from build123d import *

# Parameters (mm, degrees)
F1_DEPTH = 48
F3_DEPTH = 20
F4_T     = 1.5


# Not quite as in the source:
# - a shell that OpenCascade refuses in one call is made with other operations: the cavity is built on its own and cut out


with BuildPart() as f1:
    # F0 (on Top) → F1 (new body)
    with BuildSketch(Plane.XY):
        Polygon((22.5, 22.8382229426), (-22.5, 22.8382229426), (-25, -9.1617770574), (25, -9.1617770574), align=None)
        Polygon((19, 39.8382229426), (-19, 39.8382229426), (-22.5, 22.8382229426), (22.5, 22.8382229426), align=None)
    extrude(amount=F1_DEPTH)

    # F2 (on face) → F3 (cut)
    with BuildSketch(Plane.XY.offset(48)):
        Polygon((22.5, 22.8382229426), (-22.5, 22.8382229426), (-25, -9.1617770574), (25, -9.1617770574), align=None)
    extrude(amount=-F3_DEPTH, mode=Mode.SUBTRACT)

    # F4: shell of thickness 1.5, made by hand


with BuildPart() as f4_core1:
    # F4_t2: copy of F1
    add(f1.part)

    # the walls: a layer under each face that stays
    f4_faces = [f4_core1.faces().sort_by_distance(p)[0] for p in [
        (0, 15.3382229426, 0),
        (23.75, 6.8382229426, 14),
        (-23.75, 6.8382229426, 14),
        (20.75, 31.3382229426, 24),
        (0, 39.8382229426, 24),
        (-20.75, 31.3382229426, 24),
        (0, 31.3382229426, 48),
    ]]
    thicken(f4_faces, amount=-F4_T, mode=Mode.SUBTRACT)


with BuildPart() as f1_1:
    add(f1.part)

    # what is left inside the walls is the cavity
    f4_cavity = [f4_core1.part.solids().sort_by_distance(p)[0] for p in [
        (0, 6.671556, 1.515),
    ]]
    add(f4_cavity, mode=Mode.SUBTRACT)


solid = f1_1.part
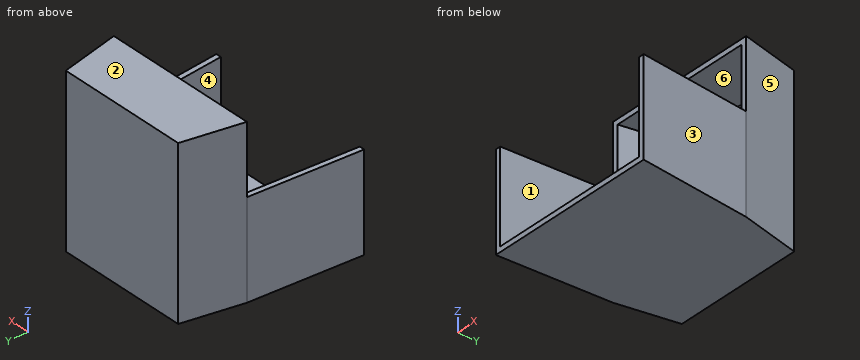
Could you check a few things on this model? Use its own coordinates, in mm. Face numbers are marked on the shaded views. A direction names the side the tool comes from. Give positions to 0.01 mm unless a question says otherwise; leave off trailing zeros. Write each loop counter-clockwise with the first axis right and the second up, starting at its lowest first coordinate (ties: lowest second). Pieces come first, ordered by that corner, then holes. Notation, with made-up numbers: (-39.5, 3) -> (-24.5, 3) arc R29 ccw to (-24.5, 23) -> close; hole circle Ø10 at (-3, 22). An arc over 180 degrees is marked (long way). Write each question's results on one line, items separated by ' | '. Start each with the question number.
Q1. Suppose I cut it at D-D, the plane y = 14. List the corners of the cut face in (x, z) for me.
Q2. Suppose I cut it at A-A, the plane x = -7. List the corners of the cut face in (y, z) for me, and give its area (4 significant figures).
Q3. Suppose I cut it at B-B, the plane y = 28.5. List the corners of the cut face in (x, z) for me, and give its area (3 significant figures).
Q4. Suppose I cut it at C-C, the plane z = 18. List the corners of the cut face in (x, y) for me, and give its area (3 significant figures).
Q5. Which directions (+Z, -Z, +X, -X, +Y, -Y) give clear straight access to the entire face, cutting with the end or side of a thin tool? Please do the marked faces 5 and 6.
Q6. We'd pull the mould along X, two halves only. Please class the marked faces 1, 2, 3 and 4: +X half, -X half, draft (parallel to the pull), parting line (faces both ways), or undercut.
Q7. I'm going to push flat-ended pins straight in: pin 1 Ø3 at (x, z) = (8, 33.5) entering from -Y; pin 2 Ø3 at (x, y) = (22.5, 14) entering from +Z; pin 3 Ø22 at (x, z) = (1.5, 38) entering from -Y. Where does each tip first touch, or does it pass through?
Q8. I need wall thicknesses on probe 1 along Z at (x, y) = (0, 35); probe 2 along Y at (x, z) = (-15, 31.5); probe 3 along X at (y, z) = (34.5, 23.5). Which ranges of each line are inside material? Lowest first, please.
Outcome:
1) outline: (-23.19, 0) -> (23.19, 0) -> (23.19, 28) -> (21.69, 28) -> (21.69, 1.5) -> (-21.69, 1.5) -> (-21.69, 28) -> (-23.19, 28) -> close
2) outline: (-9.16, 0) -> (39.84, 0) -> (39.84, 48) -> (22.84, 48) -> (22.84, 46.5) -> (38.34, 46.5) -> (38.34, 1.5) -> (-9.16, 1.5) -> close | area: 166.5 mm2
3) outline: (-21.33, 0) -> (21.33, 0) -> (21.33, 48) -> (-21.33, 48) -> close; hole (-19.8, 1.5) -> (19.8, 1.5) -> (19.8, 46.5) -> (-19.8, 46.5) -> close | area: 266 mm2
4) outline: (-25, -9.16) -> (-23.5, -9.16) -> (-21.01, 22.63) -> (-17.78, 38.34) -> (17.78, 38.34) -> (21.01, 22.63) -> (23.5, -9.16) -> (25, -9.16) -> (22.5, 22.84) -> (19, 39.84) -> (-19, 39.84) -> (-22.5, 22.84) -> close | area: 201 mm2
5) face 5: +Z, -Z, +X, +Y | face 6: -Y
6) face 1: undercut | face 2: draft | face 3: +X half | face 4: undercut
7) pin 1: y = 38.34 | pin 2: z = 28 | pin 3: y = 22.84
8) probe 1: 0 to 1.5, 46.5 to 48 | probe 2: 38.34 to 39.84 | probe 3: -20.1 to -18.57, 18.57 to 20.1
